Verification items for the finished model (mm, model axes). Face numbers are marked on the shaded views. Coordinates: 2 decimals unless noted, no trailing zeros. Order: outer loops, then holes, each group sorted by start corner. A loop starts at its lowest first (then second) coordinate and runs counter-clockwise, first axis right, second up. Notation, with made-up numbers: M 61,50 L 112,50 A26 ccw 112,72 Z; hole C 71,11.25 d6. An arc over 180 degrees is marked long. Return JSON: item names as keys, results as strings.
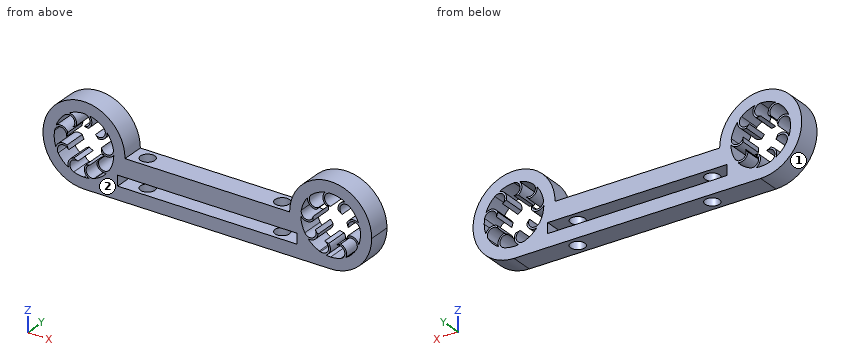
```python
from build123d import *

# Parameters (mm, degrees)
F1_DEPTH = 5
F3_DEPTH = 5
F4_W     = 5
F4_H     = 2.3
F5_DEPTH = 20
F6_R     = 1.6
F7_DEPTH = 18.301


# Not quite as in the source:
# - a pattern or mirror of a feature is missing from the dataset's text; its kind, count and spacing are read off the source's solid


with BuildPart() as f1:
    # F0 (on Front) → F1 (new body)
    with BuildSketch(Plane.XZ):
        with BuildLine():
            ThreePointArc((-27.5, -15.6002467841), (-32.2022600949, -4.2479866892), (-20.85, -8.9502467841))
            Line((-20.85, -8.9502467841), (-18.35, -8.9502467841))
            ThreePointArc((-18.35, -8.9502467841), (-33.9700270479, -2.4802197362), (-27.5, -18.1002467841))
            Line((-27.5, -18.1002467841), (-27.5, -15.6002467841))
        make_face()
        with BuildLine():
            Line((-18.35, -8.9502467841), (-20.85, -8.9502467841))
            Line((-20.85, -8.9502467841), (-20.85, -15.1002467841))
            Line((-20.85, -15.1002467841), (-20.7250461256, -15.1002467841))
            ThreePointArc((-20.7250461256, -15.1002467841), (-18.9643884826, -12.2465835425), (-18.35, -8.9502467841))
        make_face()
        with BuildLine():
            ThreePointArc((-24.9701778719, -15.1002467841), (-26.2106203042, -15.4740493562), (-27.5, -15.6002467841))
            Line((-27.5, -15.6002467841), (-27.5, -18.1002467841))
            ThreePointArc((-27.5, -18.1002467841), (-23.7952732894, -17.3166976445), (-20.7250461256, -15.1002467841))
            Line((-20.7250461256, -15.1002467841), (-20.85, -15.1002467841))
            Line((-20.85, -15.1002467841), (-24.9701778719, -15.1002467841))
        make_face()
        with BuildLine():
            Line((18.35, -8.9502467841), (-18.35, -8.9502467841))
            ThreePointArc((-18.35, -8.9502467841), (-18.9643884826, -12.2465835425), (-20.7250461256, -15.1002467841))
            Line((-20.7250461256, -15.1002467841), (20.7250461256, -15.1002467841))
            ThreePointArc((20.7250461256, -15.1002467841), (18.9643884826, -12.2465835425), (18.35, -8.9502467841))
        make_face()
        with BuildLine():
            ThreePointArc((-20.7250461256, -15.1002467841), (-23.7952732894, -17.3166976445), (-27.5, -18.1002467841))
            Line((-27.5, -18.1002467841), (27.5, -18.1002467841))
            ThreePointArc((27.5, -18.1002467841), (23.7952732894, -17.3166976445), (20.7250461256, -15.1002467841))
            Line((20.7250461256, -15.1002467841), (-20.7250461256, -15.1002467841))
        make_face()
        with BuildLine():
            Line((20.85, -8.9502467841), (18.35, -8.9502467841))
            ThreePointArc((18.35, -8.9502467841), (18.9643884826, -12.2465835425), (20.7250461256, -15.1002467841))
            Line((20.7250461256, -15.1002467841), (20.85, -15.1002467841))
            Line((20.85, -15.1002467841), (20.85, -8.9502467841))
        make_face()
        with BuildLine():
            ThreePointArc((36.65, -8.9502467841), (27.5, 0.1997532159), (18.35, -8.9502467841))
            Line((18.35, -8.9502467841), (20.85, -8.9502467841))
            ThreePointArc((20.85, -8.9502467841), (27.5, -2.3002467841), (34.15, -8.9502467841))
            ThreePointArc((34.15, -8.9502467841), (32.2022600949, -13.652506879), (27.5, -15.6002467841))
            Line((27.5, -15.6002467841), (27.5, -18.1002467841))
            ThreePointArc((27.5, -18.1002467841), (33.9700270479, -15.4202738319), (36.65, -8.9502467841))
        make_face()
        with BuildLine():
            ThreePointArc((20.7250461256, -15.1002467841), (23.7952732894, -17.3166976445), (27.5, -18.1002467841))
            Line((27.5, -18.1002467841), (27.5, -15.6002467841))
            ThreePointArc((27.5, -15.6002467841), (26.2106203042, -15.4740493562), (24.9701778719, -15.1002467841))
            Line((24.9701778719, -15.1002467841), (20.85, -15.1002467841))
            Line((20.85, -15.1002467841), (20.7250461256, -15.1002467841))
        make_face()
        with BuildLine():
            Line((-20.85, -15.1002467841), (-20.85, -8.9502467841))
            ThreePointArc((-20.85, -8.9502467841), (-21.9752458357, -12.6515426955), (-24.9701778719, -15.1002467841))
            Line((-24.9701778719, -15.1002467841), (-20.85, -15.1002467841))
        make_face()
        with BuildLine():
            ThreePointArc((24.9701778719, -15.1002467841), (21.9752458357, -12.6515426955), (20.85, -8.9502467841))
            Line((20.85, -8.9502467841), (20.85, -15.1002467841))
            Line((20.85, -15.1002467841), (24.9701778719, -15.1002467841))
        make_face()
    extrude(amount=F1_DEPTH)

    # F2 (on face) → F3 (join, through all)
    with BuildSketch(Plane(origin=(0, 0, 0), x_dir=(-1, 0, 0), z_dir=(0, 1, 0))):
        with BuildLine():
            ThreePointArc((27.5, -5.0002467841), (26.15, -3.6502467841), (27.5, -2.3002467841))
            ThreePointArc((27.5, -2.3002467841), (26.8763316072, -2.3295566587), (26.2581608513, -2.4172279162))
            ThreePointArc((26.2581608513, -2.4172279162), (25.7598479988, -3.8356409932), (26.5458163918, -5.1172279162))
            ThreePointArc((26.5458163918, -5.1172279162), (27.0193361509, -5.0296011403), (27.5, -5.0002467841))
        make_face()
        with BuildLine():
            ThreePointArc((24.9609889417, -5.9243712338), (23.0590656705, -5.7579745086), (23.2254623956, -3.8560512373))
            ThreePointArc((23.2254623956, -3.8560512373), (22.7665447132, -4.2793902194), (22.3493524387, -4.7439028016))
            ThreePointArc((22.3493524387, -4.7439028016), (22.8793609985, -6.1507795846), (24.3052359132, -6.6273213807))
            ThreePointArc((24.3052359132, -6.6273213807), (24.6116476876, -6.2558227419), (24.9609889417, -5.9243712338))
        make_face()
        with BuildLine():
            ThreePointArc((23.6100093756, -8.2643364823), (22.0460938692, -9.359401909), (20.9510284425, -7.7954864026))
            ThreePointArc((20.9510284425, -7.7954864026), (20.8715941544, -8.4147694774), (20.8505892632, -9.0387727847))
            ThreePointArc((20.8505892632, -9.0387727847), (22.1609223396, -9.7758199912), (23.5595210567, -9.2243374579))
            ThreePointArc((23.5595210567, -9.2243374579), (23.5554513717, -8.742795298), (23.6100093756, -8.2643364823))
        make_face()
        with BuildLine():
            ThreePointArc((21.7409310648, -12.2752467841), (22.0781483573, -12.8007045184), (22.4631592713, -13.2922204683))
            ThreePointArc((22.4631592713, -13.2922204683), (23.9406974553, -13.014565519), (24.6576000913, -11.6931034626))
            ThreePointArc((24.6576000913, -11.6931034626), (24.3449531978, -11.32683671), (24.0791996551, -10.9252467841))
            ThreePointArc((24.0791996551, -10.9252467841), (23.5850653599, -12.7693810792), (21.7409310648, -12.2752467841))
        make_face()
        with BuildLine():
            ThreePointArc((25.2255660469, -15.1992027123), (25.8216472009, -15.3849675925), (26.4325230347, -15.5140104094))
            ThreePointArc((26.4325230347, -15.5140104094), (27.3859097889, -14.3515711409), (27.0856696329, -12.878456344))
            ThreePointArc((27.0856696329, -12.878456344), (26.6107364871, -12.7988452828), (26.1490204339, -12.6620326362))
            ThreePointArc((26.1490204339, -12.6620326362), (26.9558782784, -14.3923448677), (25.2255660469, -15.1992027123))
        make_face()
        with BuildLine():
            ThreePointArc((29.7744339531, -15.1992027123), (30.3504659721, -14.9583532863), (30.9013711338, -14.6645424021))
            ThreePointArc((30.9013711338, -14.6645424021), (30.8845062002, -13.1612370672), (29.7076089581, -12.2257563152))
            ThreePointArc((29.7076089581, -12.2257563152), (29.2926160571, -12.4700518457), (28.8509795661, -12.6620326362))
            ThreePointArc((28.8509795661, -12.6620326362), (30.5812917977, -13.4688904808), (29.7744339531, -15.1992027123))
        make_face()
        with BuildLine():
            ThreePointArc((33.2590689352, -12.2752467841), (33.5455200355, -11.7204791751), (33.7786798774, -11.1412919678))
            ThreePointArc((33.7786798774, -11.1412919678), (32.7994545459, -10.0005338401), (31.2965835169, -10.0404089735))
            ThreePointArc((31.2965835169, -10.0404089735), (31.1357106513, -10.494302502), (30.9208003449, -10.9252467841))
            ThreePointArc((30.9208003449, -10.9252467841), (32.7649346401, -10.431112489), (33.2590689352, -12.2752467841))
        make_face()
        with BuildLine():
            ThreePointArc((31.3899906244, -8.2643364823), (32.4850560511, -6.7004209759), (34.0489715575, -7.7954864026))
            ThreePointArc((34.0489715575, -7.7954864026), (33.9118080859, -7.1863825404), (33.7181245266, -6.5928271413))
            ThreePointArc((33.7181245266, -6.5928271413), (32.2347292126, -6.3483896268), (31.1090944539, -7.3449626276))
            ThreePointArc((31.1090944539, -7.3449626276), (31.2776158253, -7.7960723276), (31.3899906244, -8.2643364823))
        make_face()
        with BuildLine():
            ThreePointArc((30.0390110583, -5.9243712338), (29.8726143331, -4.0224479625), (31.7745376044, -3.8560512373))
            ThreePointArc((31.7745376044, -3.8560512373), (31.2779398735, -3.4776175885), (30.748039603, -3.1474251655))
            ThreePointArc((30.748039603, -3.1474251655), (29.4545714601, -3.9136832939), (29.2328699852, -5.4006465792))
            ThreePointArc((29.2328699852, -5.4006465792), (29.6519325712, -5.6378932086), (30.0390110583, -5.9243712338))
        make_face()
    f3 = extrude(amount=-F3_DEPTH)

    # F3_copies: F3 across plane
    add(f3.mirror(Plane(origin=(0, 0, 0), x_dir=(0, 0, 1), z_dir=(1, 0, 0))))

    # F4 (on Right) → F5 (cut, symmetric)
    with BuildSketch(Plane.YZ):
        with Locations((-2.5, -14.0502467841)):
            Rectangle(F4_W, F4_H)
    extrude(amount=F5_DEPTH, both=True, mode=Mode.SUBTRACT)

    # F6 (on face) → F7 (cut, through all)
    with BuildSketch(Plane(origin=(0, 0, -18.1002467841), x_dir=(1, 0, 0), z_dir=(0, 0, -1))):
        with Locations((-15, 2.5)):
            Circle(F6_R)
        with Locations((15, 2.5)):
            Circle(F6_R)
    extrude(amount=-F7_DEPTH, mode=Mode.SUBTRACT)


solid = f1.part
```
Q1. Cross-section at C-C, the plane y = -2.5. State how many separate pieces and enclosed holes the cut face has, and give its area (3 significant figures).
Values:
{"separate pieces": "4", "enclosed holes": "2", "area": "508 mm^2"}
Q2. Cross-section at A-A, the plane x = 15. Record the boundary of the cut face in (y, z), and give its area (3 significant figures).
Values:
{"outline": "M -5,-18.1 L -4.1,-18.1 L -4.1,-15.2 L -5,-15.2 Z; M -5,-12.9 L -4.1,-12.9 L -4.1,-8.95 L -5,-8.95 Z; M -0.9,-18.1 L 0,-18.1 L 0,-15.2 L -0.9,-15.2 Z; M -0.9,-12.9 L 0,-12.9 L 0,-8.95 L -0.9,-8.95 Z", "area": "12.3 mm^2"}
Q3. Draft check along X on the marked faces 1 and 2. Enter one of: pulls with the +X half, pulls with the -X half, needs draft (parallel to the pull), parting line crosses it, or undercut.
Values:
{"face 1": "undercut", "face 2": "needs draft"}
Q4. Go/stop test with flat-tipped pins: pin 1 (1.5 mm diameter, centred on x = -0.5, y = -3, fed in from +Z); pin 2 (1.2 mm diameter, centred on y = -3.5, z = -13.5, fed in from -X); pin 3 (1.8 mm diameter, centred on y = -3, z = -14.5, fed in from +X); pin 4 (3 mm diameter, centred on x = 15, y = -2.5, fed in from -Z). Record where each tip stops, or that it passes through.
Values:
{"pin 1": "z = -8.95", "pin 2": "x = -35.75", "pin 3": "x = 35.38", "pin 4": "through"}
Q5. Material ranges on line 1 along Y through (x, z) = (-15, -16.8); line 2 along Z through (x, y) = (-22, -4.1); line 3 along Z through (x, y) = (-24, -2.4), recorded low to high.
Values:
{"line 1": "-5 to -4.1, -0.9 to 0", "line 2": "-18.1 to -12.6, -9.76 to -9.35, -5.21 to -1.64", "line 3": "-18.1 to -14.6, -12.97 to -12.4, -6.64 to -6.24, -3.3 to -0.5"}
Q6. Cross-section at B-B, the plane x = -0.5. Record the boundary of the cut face in (y, z), and give its area (4 significant figures).
Values:
{"outline": "M -5,-18.1 L 0,-18.1 L 0,-15.2 L -5,-15.2 Z; M -5,-12.9 L 0,-12.9 L 0,-8.95 L -5,-8.95 Z", "area": "34.25 mm^2"}
